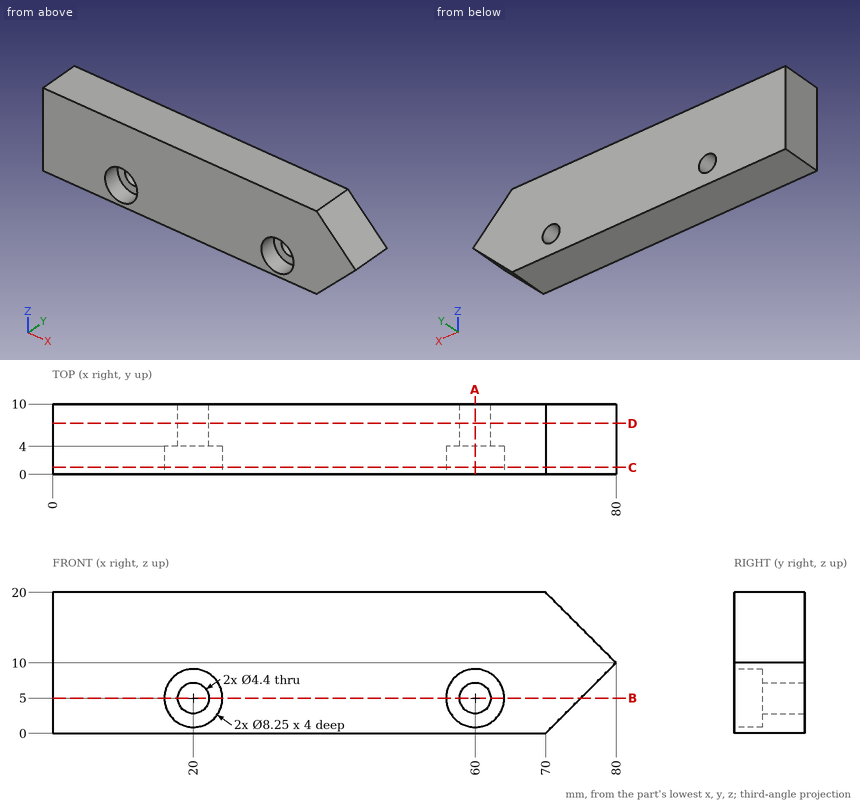
Geometry check sheet. Reference: drawing and pictorial views, mm from the part's lowest x, y, z. Coordinates: 2 decimals unless noted, no trailing zeros. Order: outer loops, then holes, each group sorted by start corner. A loop starts at its lowest first (then second) coordinate and runs counter-clockwise, first axis right, second up.
Item 1: Material ranges on L1, parallel to Z at x = 60, y = 2.9 (3 decimals); L2, parallel to Z at x = 20, y = 6.55; L3, parallel to Y at x = 16, z = 4.5, recorded low to high.
Filled in:
L1: z = 0 to 0.875, 9.125 to 20
L2: z = 0 to 2.8, 7.2 to 20
L3: y = 4 to 10
Item 2: Section check A-A, the plane x = 60. Enter the section's corners in (y, z) (3 decimals).
Filled in:
outline: (0, 0) - (10, 0) - (10, 2.8) - (4, 2.8) - (4, 0.875) - (0, 0.875) - close; (0, 9.125) - (4, 9.125) - (4, 7.2) - (10, 7.2) - (10, 20) - (0, 20) - close
Item 3: Section check D-D, the plane y = 7.25. Enter the section's corners in (x, z), then the cut area to 3 significant figures.
Filled in:
outline: (0, 0) - (70, 0) - (80, 10) - (70, 20) - (0, 20) - close; hole circle Ø4.4 at (20, 5); hole circle Ø4.4 at (60, 5)
area: 1,470 mm2
Item 4: Section check B-B, the plane z = 5. Enter the section's corners in (x, y) (3 decimals), then the cut area to 3 significant figures.
Filled in:
outline: (0, 0) - (15.875, 0) - (15.875, 4) - (17.8, 4) - (17.8, 10) - (0, 10) - close; (22.2, 4) - (24.125, 4) - (24.125, 0) - (55.875, 0) - (55.875, 4) - (57.8, 4) - (57.8, 10) - (22.2, 10) - close; (62.2, 4) - (64.125, 4) - (64.125, 0) - (75, 0) - (75, 10) - (62.2, 10) - close
area: 631 mm2
Item 5: Section check C-C, the plane y = 1. Enter the section's corners in (x, z) (3 decimals).
Filled in:
outline: (0, 0) - (70, 0) - (80, 10) - (70, 20) - (0, 20) - close; hole circle Ø8.25 at (20, 5); hole circle Ø8.25 at (60, 5)
Item 6: Depth check by flat-ended pin: pin 1 (5 mm diameter, centred on x = 20, z = 5, fed in from -Y); pin 2 (5 mm diameter, centred on y = 5.5, z = 2.5, fed in from +X). Enter the tip coordinate at first touch or a pass-through.
Filled in:
pin 1: stops at y = 4
pin 2: stops at x = 75
